```python
from build123d import *

# Parameters (mm, degrees)
PAD_DEPTH    = 60
SKETCH001_R  = 3
PAD001_DEPTH = 60
FILLET_R     = 1
FILLET001_R  = 1


with BuildPart() as part:
    # Sketch → Pad (new body)
    with BuildSketch(Plane.XZ):
        with BuildLine():
            ThreePointArc((-4, -3), (0, -5), (4, -3))
            Line((4, -3), (6.324555, -3))
            ThreePointArc((6.324555, -3), (0, 7), (-6.324555, -3))
            Line((-4, -3), (-6.324555, -3))
        make_face()
    extrude(amount=PAD_DEPTH)

    # Sketch001 → Pad001 (join)
    with BuildSketch(Plane.XZ):
        Circle(SKETCH001_R)
    extrude(amount=-PAD001_DEPTH)

    # Fillet
    fillet_edges = [part.edges().sort_by_distance(p)[0] for p in [
        (0, 0, 7),
        (0, 0, -5),
    ]]
    fillet(fillet_edges, radius=FILLET_R)

    # Fillet001
    fillet001_edges = [part.edges().sort_by_distance(p)[0] for p in [
        (-3, 60, 0),
    ]]
    fillet(fillet001_edges, radius=FILLET001_R)


solid = part.part
```
For this review, take the finished solid that the model builds, in its own axes (mm). A direction names the side the tool comes from. Coordinates: 2 decimals unless noted, no trailing zeros. Write each loop counter-clockwise with the first axis right and the second up, starting at its lowest first coordinate (ties: lowest second). Pieces come first, ordered by that corner, then holes. Notation, with made-up numbers: (25, -24.75) - (34, -24.75) arc R22 ccw to (34, -11.75) - close; hole circle Ø5 at (63.25, 59). An arc over 180 degrees is marked (long way). Put each result on its own line as item: value.
1. For pin 1 (1 mm diameter, centred on x = -3, y = 41, fed in from -Z); pin 2 (1.1 mm diameter, centred on x = -5, y = -34, fed in from -Z); pin 3 (2 mm diameter, centred on y = 44.5, z = 2, fed in from -X), all flat-tipped, find the tip position at first contact; note any pin that passes through.
Values found:
pin 1: z = -1.66
pin 2: z = -3
pin 3: x = -2.83
2. Machinability: for faces 1 (the cylindrical face through (0, -30, -5)), 2 (the cylindrical face through (-3, 29, 0)), which of the approach directions +Z, -Z, +X, -X, +Y, -Y give a long, thin tool a straight path to every point of the face, cutting with its end or side? Answer none if there is none.
Values found:
face 1: -Z, +Y, -Y
face 2: +Y
3. Add section A-A, the plane x = 0. Give the boundary of the cut face in (y, z), then the cut area to 3 significant figures.
Values found:
outline: (-60, -5) - (-1, -5) arc R1 ccw to (0, -4) - (0, -3) - (59, -3) arc R1 ccw to (60, -2) - (60, 2) arc R1 ccw to (59, 3) - (0, 3) - (0, 6) arc R1 ccw to (-1, 7) - (-60, 7) - close
area: 1,080 mm²
4. Wall thickness on probe 1 along Y at (x, z) = (0, -3.5); probe 2 along Z at (x, y) = (3, -12); probe 3 along Y at (x, z) = (-4.5, 5): over which ranges is each line inside the solid? List them lowest first.
Values found:
probe 1: -60 to 0
probe 2: -4 to 6.32
probe 3: -60 to -0.31
5. Add section B-B, the plane y = -20.5. Give the boundary of the cut face in (x, z), then the cut area to 3 significant figures.
Values found:
outline: (-6.32, -3) - (-4, -3) arc R5 ccw to (4, -3) - (6.32, -3) arc R7 ccw (long way) to start
area: 129 mm²
